Check sheet for the modelled part. Datum: model origin and axes. Units: mm. A direction names the side the tool comes from. Give positions to 0.01 mm unless a question says otherwise; leave off trailing zeros. Put each result on its own line as item: value. Start each with the question number.
```python
from build123d import *
from OCP.BRepFilletAPI import BRepFilletAPI_MakeChamfer

# Parameters (mm, degrees)
SKETCH1_R           = 22.25
BOSS_EXTRUDE1_DEPTH = 6
FILLET1_R           = 1
SKETCH3_R           = 12.695
CUT_EXTRUDE1_DEPTH  = 92.957544552
CHAMFER1_SIZE       = 0.5
CHAMFER1_SIZE2      = 0.523325215
BOSS_EXTRUDE2_DEPTH = 20
CHAMFER2_SIZE       = 3.5
FILLET2_R           = 1


with BuildPart() as part:
    # Sketch1 → Boss-Extrude1 (new body)
    with BuildSketch(Plane.XY):
        Circle(SKETCH1_R)
    extrude(amount=BOSS_EXTRUDE1_DEPTH)

    # Sketch2 → Revolve1 (revolve)
    with BuildSketch(Plane(origin=(0, 0, 0), x_dir=(1, 0, 0), z_dir=(0, 1, 0))):
        Polygon((-14.5, -12.508403374), (-14.5, -33.7), (0, -33.7), (0, -6), (-60.5, -6), (-60.5, -10.5), align=None)
    revolve(axis=Axis((0, 0, 33.7), (0, 0, 1)))

    # Fillet1
    fillet1_edges = [part.edges().sort_by_distance(p)[0] for p in [
        (-22.25, 0, 6),
    ]]
    fillet(fillet1_edges, radius=FILLET1_R)

    # Sketch3 → Cut-Extrude1 (cut, through all)
    with BuildSketch(Plane.XY.offset(33.7)):
        Circle(SKETCH3_R)
    extrude(amount=-CUT_EXTRUDE1_DEPTH, mode=Mode.SUBTRACT)

    # Chamfer1: one chamfer whose edges measure the first distance from different faces: ONE call of the kernel's chamfer builder (chamfer() names one face for all edges)
    chamfer1_edges_1 = [part.edges().sort_by_distance(p)[0] for p in [
        (-22.25, 0, 0),
        (60.5, 0, 6),
        (14.5, 0, 33.7),
    ]]
    chamfer1_edges_2 = [part.edges().sort_by_distance(p)[0] for p in [
        (60.5, 0, 10.5),
    ]]
    chamfer1_side_2 = [part.faces().sort_by_distance(p)[0] for p in [
        (37.5, 0, 11.504201687),
    ]]
    chamfer1 = BRepFilletAPI_MakeChamfer(part.part.solid().wrapped)
    for e in chamfer1_edges_1:
        chamfer1.Add(CHAMFER1_SIZE, e.wrapped)
    for e in chamfer1_edges_2:
        chamfer1.Add(CHAMFER1_SIZE, CHAMFER1_SIZE2, e.wrapped, chamfer1_side_2[0].wrapped)  # the first distance lies on this face
    add(Compound.cast(chamfer1.Shape()), mode=Mode.REPLACE)

    # Sketch4 → Boss-Extrude2 (add)
    with BuildSketch(Plane.XY.offset(33.7)):
        with BuildLine():
            Line((-3.075, -12.316955793), (-3.075, -9.61))
            Line((-3.075, -9.61), (3.075, -9.61))
            Line((3.075, -9.61), (3.075, -12.316955793))
            ThreePointArc((3.075, -12.316955793), (0, -12.695), (-3.075, -12.316955793))
        make_face()
    extrude(amount=-BOSS_EXTRUDE2_DEPTH)

    # Sketch5 → Cut-Revolve1 (revolve, cut)
    with BuildSketch(Plane(origin=(0, 0, 0), x_dir=(1, 0, 0), z_dir=(0, 1, 0)), mode=Mode.PRIVATE) as cut_revolve1_sk:
        Polygon((-12.695, -33.2), (-13.195, -33.7), (-12.695, -33.7), align=None)
        Polygon((-9.195, -33.7), (-12.695, -33.7), (-12.695, -33.2), (-9.195, -29.7), align=None)
    revolve(cut_revolve1_sk.sketch.rotate(Axis((0, 0, 0), (0, 0, -1)), 180), axis=Axis((0, 0, 0), (0, 0, -1)), mode=Mode.SUBTRACT)

    # Chamfer2
    # the kernel refuses this chamfer: 3.5 mm, written as the material it takes off along each edge
    with BuildSketch(Plane(origin=(-12.075890458, -9.61, 13.7), x_dir=(0, -0.9996219169112968, -0.027495876610586605), z_dir=(1, 0, 0))) as chamfer2_piece_1_section:
        Polygon((CHAMFER2_SIZE * 0.999621916911, -CHAMFER2_SIZE * 0.0274958766106), (-CHAMFER2_SIZE * 0.0274958766106, -CHAMFER2_SIZE * 0.999621916911), (0, 0), align=None)
    chamfer2_piece_1 = extrude(amount=24.151780916, mode=Mode.PRIVATE)
    chamfer2_piece_1 = chamfer2_piece_1 & Plane(origin=(0, 0, 14.984613596), x_dir=(1, 0, 0), z_dir=(0, 0, 1)) * Cylinder(12.695, 63, mode=Mode.PRIVATE)
    add(chamfer2_piece_1, mode=Mode.SUBTRACT)

    # Fillet2
    fillet2_edges = [part.edges().sort_by_distance(p)[0] for p in [
        (14.5, 0, 12.508403374),
    ]]
    fillet(fillet2_edges, radius=FILLET2_R)


solid = part.part
```
Q1. Depth check by flat-ended pin: P1, Ø6, axis at y = 35, z = 10.5, coming from the +X side; P2, Ø1.8, axis at x = 0, z = 22, coming from the +Y side; P3, Ø0.8, axis at y = -11, z = 23.5, coming from the +X side; P4, Ø6, axis at y = 37, z = 17, coming from the -X side. Enter the tip coordinate at first touch or a pass-through.
Q2. Mould release check, pull along X, two halves, no side actions. Record for faces 1 (the face through (-3.075, -11, 24)), 2 (the face through (13.12, 59.06, 8.26)), 3 (the face through (-1, 26, 6)): pulls with the +X half, pulls with the -X half, needs draft (parallel to the pull), parting line crosses it, or undercut.
Q3. Thickness scan on line 1 along X through (y, z) = (0, 26) (3 decimals); line 2 along Y through (x, z) = (0, 10) (3 decimals); line 3 along Y through (x, z) = (0, 22) (3 decimals). Record the ranges inside material, lowest first. Write a range as [from, to].
Q4. Access from +Z, -Z, +X, -X, +Y, -Y to the whole of each face (thin tool, end or side, straight path). Record for faces 4 (the face through (-16.399, 15.038, 2.718)), 5 (the face through (0, -9.61, 24)), 6 (the face through (3.143, 14.155, 23.471)).
Found:
1. P1: stops at x = 51.32
1. P2: stops at y = 14.5
1. P3: stops at x = 9.89
1. P4: passes through
2. face 1: undercut
2. face 2: parting line crosses it
2. face 3: needs draft
3. line 1: x = [-14.5, -12.695], [12.695, 14.5]
3. line 2: y = [-60.479, -12.695], [12.695, 60.479]
3. line 3: y = [-14.5, -9.61], [12.695, 14.5]
4. face 4: -Z
4. face 5: +Z, -Z
4. face 6: +Z
